Read the model definition and answer for the solid it produces. Units are mm, in the model's axes. Face numbers are marked on the shaded views. A direction names the side the tool comes from. Round coordinates to 2 decimals unless told otherwise and drop trailing zeros. Write each loop counter-clockwise with the first axis right and the second up, starting at its lowest first coordinate (ties: lowest second). Pieces come first, ordered by that corner, then holes. Notation, with made-up numbers: (-11.75, 45.25) - (31.25, 45.25) arc R14 ccw to (31.25, 59.25) - close; hole circle Ø8 at (46, 13). An arc over 180 degrees is marked (long way). Answer as CSV lines item,"result". Start each with the question number.
1) Which of the six approach directions +Z, -Z, +X, -X, +Y, -Y give full straight-line access (tool end or side, diameter ignored) to the marked faces 5 and 6?
2) Find section C-C on y = 3.5. Determine the outline of the cut face in (x, z), then the cut area to 3 significant figures.
3) Find section A-A on z = 0. Determine the outline of the cut face in (x, y), then the cut area to 3 significant figures.
4) Consider line 1 along Z through (x, y) = (10.44, 5.25); line 2 along X through (y, z) = (2.75, 0); line 3 along X through (y, z) = (5.25, 0.25). Determine where each line is inside the solid, lowest interval first.
5) For a pull along X with two mould halves and no side action, classify the marked faces 1, 2, 3 and 4 as +X half, -X half, draft (parallel to the pull), parting line (faces both ways), or undercut.
6) Find section D-D on z = -2. Determine the outline of the cut face in (x, y), then the cut area to 3 significant figures.
7) Find section B-B on x = -8.44. Determine the outline of the cut face in (y, z), then the cut area to 4 significant figures.
from build123d import *

# Parameters (mm, degrees)
SKETCH1_W               = 25
SKETCH1_H               = 7
SKETCH1_R               = 1.75
BOSS_EXTRUDE1_DEPTH     = 6.5
CUT_EXTRUDE1_DEPTH      = 15.517231141
CUT_EXTRUDE1_DEPTH_BACK = 15.517231141


with BuildPart() as part:
    # Sketch1 → Boss-Extrude1 (new body)
    with BuildSketch(Plane(origin=(0, 0, 0), x_dir=(1, 0, 0), z_dir=(0, 1, 0))):
        Rectangle(SKETCH1_W, SKETCH1_H)
        with Locations(Location((10.44, 0, 0), (0, 0, 90))):
            Circle(SKETCH1_R, mode=Mode.SUBTRACT)
        with Locations(Location((-8.44, 0, 0), (0, 0, 90))):
            Circle(SKETCH1_R, mode=Mode.SUBTRACT)
    extrude(amount=BOSS_EXTRUDE1_DEPTH)

    # Sketch3 → Cut-Extrude1 (cut, two sides: drawn at the far end of the back side and taken through both)
    with BuildSketch(Plane.XY.offset(-CUT_EXTRUDE1_DEPTH_BACK)):
        Polygon((1.425586366, 0.076503178), (2.811602997, 2.522845597), (1.386016631, 4.946342419), (-1.425586366, 4.923496822), (-2.811602997, 2.477154403), (-1.386016631, 0.053657581), align=None)
    extrude(amount=CUT_EXTRUDE1_DEPTH + CUT_EXTRUDE1_DEPTH_BACK, mode=Mode.SUBTRACT)


solid = part.part
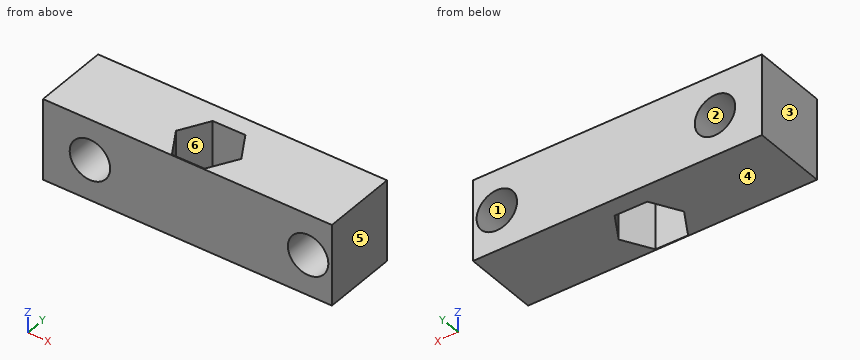
Check values:
1,face 5,"+Z, -Z, +X, +Y, -Y"
1,face 6,"+Z, -Z"
2,outline,"(-12.5, -3.5) - (-2.23, -3.5) - (-2.23, 3.5) - (-12.5, 3.5) - close; (2.24, -3.5) - (12.5, -3.5) - (12.5, 3.5) - (2.24, 3.5) - close; hole circle Ø3.5 at (-8.44, 0); hole circle Ø3.5 at (10.44, 0)"
2,area,"124 mm^2"
3,outline,"(-12.5, 0) - (-10.19, 0) - (-10.19, 6.5) - (-12.5, 6.5) - close; (-6.69, 0) - (8.69, 0) - (8.69, 6.5) - (-6.69, 6.5) - close; (12.19, 0) - (12.5, 0) - (12.5, 6.5) - (12.19, 6.5) - close; hole (-2.81, 2.48) - (-1.39, 0.05) - (1.43, 0.08) - (2.81, 2.52) - (1.39, 4.95) - (-1.43, 4.92) - close"
3,area,"96.5 mm^2"
4,line 1,"z = -3.5 to -1.75, 1.75 to 3.5"
4,line 2,"x = -12.5 to -10.19, -6.69 to -2.66, 2.68 to 8.69, 12.19 to 12.5"
4,line 3,"x = -12.5 to -10.17, -6.71 to 8.71, 12.17 to 12.5"
5,face 1,"undercut"
5,face 2,"undercut"
5,face 3,"-X half"
5,face 4,"draft"
6,outline,"(-12.5, 0) - (12.5, 0) - (12.5, 6.5) - (-12.5, 6.5) - close; hole (-2.81, 2.48) - (-1.39, 0.05) - (1.43, 0.08) - (2.81, 2.52) - (1.39, 4.95) - (-1.43, 4.92) - close"
6,area,"142 mm^2"
7,outline,"(0, -3.5) - (6.5, -3.5) - (6.5, -1.75) - (0, -1.75) - close; (0, 1.75) - (6.5, 1.75) - (6.5, 3.5) - (0, 3.5) - close"
7,area,"22.75 mm^2"
